Read the model definition and answer for the solid it produces. Units are mm, in the model's axes. Give positions to 0.01 mm unless a question says otherwise; leave off trailing zeros. Loops run counter-clockwise (first coordinate to the right, second up) from the corner with the lowest first, then second, coordinate; pieces in that order, holes last. Notation, with made-up numbers: M -30,10 L -16,10 A20 ccw -16,17 Z; hole C 45.25,-30 d11. An arc over 180 degrees is marked long. Return JSON: item names as keys, results as strings. Group by question number.
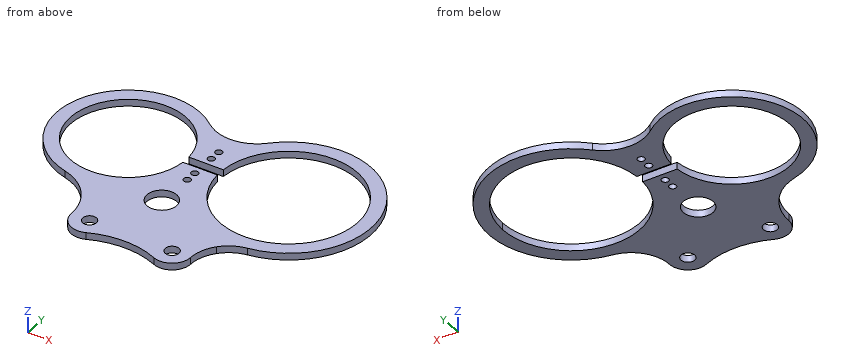
```python
from build123d import *

# Parameters (mm, degrees)
F0_R     = 4.7625
F0_R_2   = 10.31875
F0_R_3   = 2.413
F1_DEPTH = 4.7625


with BuildPart() as f1:
    # F0 (on Top) → F1 (new body)
    with BuildSketch(Plane.XY):
        with BuildLine():
            ThreePointArc((41.275, -44.45), (42.979239, -35.116466), (47.87201, -26.9875))
            Line((47.87201, -26.9875), (-45.826281, -26.9875))
            ThreePointArc((-45.826281, -26.9875), (-42.431513, -35.42707), (-41.275, -44.45))
            ThreePointArc((-41.275, -44.45), (-35.519907, -55.082886), (-23.470548, -56.07904))
            ThreePointArc((-23.470548, -56.07904), (0, -51.154707), (23.470548, -56.07904))
            ThreePointArc((23.470548, -56.07904), (35.519907, -55.082886), (41.275, -44.45))
        make_face()
        with Locations((-28.575, -44.45)):
            Circle(F0_R, mode=Mode.SUBTRACT)
        with Locations((28.575, -44.45)):
            Circle(F0_R, mode=Mode.SUBTRACT)
        with BuildLine():
            ThreePointArc((63.848057, -18.319856), (106.425851, 63.883136), (14.954093, 78.135084))
            ThreePointArc((14.954093, 78.135084), (-4.10718, 69.597202), (-23.922089, 76.2))
            ThreePointArc((-23.922089, 76.2), (-99.630791, 60.698924), (-68.038523, -9.827805))
            ThreePointArc((-68.038523, -9.827805), (-55.179287, -16.138345), (-45.826281, -26.9875))
            Line((-45.826281, -26.9875), (47.87201, -26.9875))
            ThreePointArc((47.87201, -26.9875), (55.090906, -21.236035), (63.848057, -18.319856))
        make_face()
        with Locations((-4.720613, -4.287676)):
            Circle(F0_R_2, mode=Mode.SUBTRACT)
        with Locations((-3.759988, 21.336)):
            Circle(F0_R_3, mode=Mode.SUBTRACT)
        with Locations((-3.759988, 29.337)):
            Circle(F0_R_3, mode=Mode.SUBTRACT)
        with Locations((-3.759988, 46.863)):
            Circle(F0_R_3, mode=Mode.SUBTRACT)
        with Locations((-3.759988, 54.864)):
            Circle(F0_R_3, mode=Mode.SUBTRACT)
        with BuildLine():
            ThreePointArc((-15.688707, 34.925), (-95.5625, 38.1), (-15.688707, 41.275))
            Line((-15.688707, 41.275), (8.168731, 41.275))
            ThreePointArc((8.168731, 41.275), (57.150888, 85.573435), (103.0625, 38.1))
            ThreePointArc((103.0625, 38.1), (57.150888, -9.373435), (8.168731, 34.925))
            Line((8.168731, 34.925), (-15.688707, 34.925))
        make_face(mode=Mode.SUBTRACT)
    extrude(amount=-F1_DEPTH)


solid = f1.part
```
1. Find section C-C (z = -2.2). State how many separate pieces and enclosed holes the cut face has, and give its area (3 significant figures).
2. A flat-ended cylindrical pin translates along its axis: P1, Ø2.5, axis at x = -3, z = -2, coming from the +Y side. Find the tip coordinate at first contact, or state that the pin passes through.
3. Find section A-A (x = 45.5). Write down the section's boundary in (y, z).
4. Straight lines are drawn through the part: line 1 along X through (y, z) = (65, -4.1); line 2 along Y through (x, z) = (4, -0.95) (3 decimals); line 3 along Y through (x, z) = (28, -0.6). For each, find the intervals that lie inside material, in ascending order.
5. Find section B-B (y = 74). Write down the section's boundary in (x, z), and give its area (3 significant figures).
6. Find section D-D (x = -85). Write down the section's boundary in (y, z).
Result:
{
 "1": {"separate pieces": "1", "enclosed holes": "8", "area": "10,500 mm2"},
 "2": {"P1": "stops at y = 69.81"},
 "3": {"outline": "M -30.12,-4.76 L -8.32,-4.76 L -8.32,0 L -30.12,0 Z; M 84.52,-4.76 L 94.23,-4.76 L 94.23,0 L 84.52,0 Z"},
 "4": {"line 1": "x = -97.15 to -85.17, -25.96 to 16.41, 94.71 to 105.84", "line 2": "y = -51.292 to -9.804, 1.228 to 34.925, 41.275 to 71.188", "line 3": "y = -57.14 to -49.18, -39.72 to -0.59, 76.79 to 88.02"},
 "5": {"outline": "M -89.68,-4.76 L -73.2,-4.76 L -73.2,0 L -89.68,0 Z; M -37.92,-4.76 L -20.89,-4.76 L -20.89,0 L -37.92,0 Z; M 9.82,-4.76 L 24.46,-4.76 L 24.46,0 L 9.82,0 Z; M 86.67,-4.76 L 99.87,-4.76 L 99.87,0 L 86.67,0 Z", "area": "292 mm2"},
 "6": {"outline": "M -1.73,-4.76 L 11.02,-4.76 L 11.02,0 L -1.73,0 Z; M 65.18,-4.76 L 77.93,-4.76 L 77.93,0 L 65.18,0 Z"}
}
